Work out the finished part from the listing and answer in its coordinate system (mm). A direction names the side the tool comes from. Round coordinates to 2 decimals unless told otherwise and drop trailing zeros. Loops run counter-clockwise (first coordinate to the right, second up) from the corner with the lowest first, then second, coordinate; pieces in that order, holes last. Notation, with made-up numbers: (69.5, -35.5) - (108.5, -35.5) arc R25 cw to (108.5, -15.5) - close; hole circle Ø4 at (-29.5, 84.25). An arc over 180 degrees is marked (long way). Use CSV: the item, a comma, the result in double quotes. Start each with the question number.
from build123d import *

# Parameters (mm, degrees)
BOSS_EXTRUDE1_DEPTH      = 85
BOSS_EXTRUDE1_DEPTH_BACK = 85
SKETCH1_W                = 25
SKETCH1_H                = 25
SKETCH1_W_2              = 22
SKETCH1_H_2              = 22
SKETCH2_R                = 2
CUT_EXTRUDE1_DEPTH       = 25
SKETCH3_R                = 2
CUT_EXTRUDE2_DEPTH       = 25


with BuildPart() as part:
    # Sketch1 → Boss-Extrude1 (new, two sides: drawn at the far end of the back side and taken through both)
    with BuildSketch(Plane(origin=(0, 0, 0), x_dir=(1, 0, 0), z_dir=(0, 1, 0)).offset(-BOSS_EXTRUDE1_DEPTH_BACK)):
        Rectangle(SKETCH1_W, SKETCH1_H)
        Rectangle(SKETCH1_W_2, SKETCH1_H_2, mode=Mode.SUBTRACT)
    extrude(amount=BOSS_EXTRUDE1_DEPTH + BOSS_EXTRUDE1_DEPTH_BACK)

    # Sketch2 → Cut-Extrude1 (cut)
    with BuildSketch(Plane(origin=(0, 0, -12.5), x_dir=(-1, 0, 0), z_dir=(0, 0, -1))):
        with Locations((7.5, 80)):
            Circle(SKETCH2_R)
        with Locations((7.5, 70)):
            Circle(SKETCH2_R)
        with Locations((-7.5, 80)):
            Circle(SKETCH2_R)
        with Locations((-7.5, 70)):
            Circle(SKETCH2_R)
        with Locations((7.5, 60)):
            Circle(SKETCH2_R)
        with Locations((-7.5, 60)):
            Circle(SKETCH2_R)
    cut_extrude1 = extrude(amount=-CUT_EXTRUDE1_DEPTH, mode=Mode.SUBTRACT)

    # Mirror1: Cut-Extrude1 across plane
    add(cut_extrude1.mirror(Plane.ZX), mode=Mode.SUBTRACT)

    # Sketch3 → Cut-Extrude2 (cut)
    with BuildSketch(Plane(origin=(12.5, 0, 0), x_dir=(0, 0, -1), z_dir=(1, 0, 0))):
        with Locations((5.5, 53)):
            Circle(SKETCH3_R)
        with Locations((5.5, 42)):
            Circle(SKETCH3_R)
        with Locations((-5.5, 53)):
            Circle(SKETCH3_R)
        with Locations((-5.5, 42)):
            Circle(SKETCH3_R)
    extrude(amount=-CUT_EXTRUDE2_DEPTH, mode=Mode.SUBTRACT)


solid = part.part
Item 1: This flat-tipped pin is pushed along its axis until it touches: pin 1 Ø5 at (y, z) = (53, 5.5) entering from -X. Where does it stop, or does it pass through?
Item 2: A cutting plane is placed at A-A (z = 5.5). Determine the outline of the cut face in (x, y).
Item 3: Find the intervals of material crossed by probe 1 along Y at (x, z) = (-11.5, 5.5); probe 2 along X at (y, z) = (-70, -11.8); probe 3 along Z at (x, y) = (-5.5, 68), in increasing order. Write a range as [from, to].
Item 4: The mould has two halves that part along X. Classify faces 3 (the cylindrical face through (-11.74, 54.352, -4.026)), 4 (the flat face through (12.5, -1, 0)), 5 (the cylindrical face through (-7.24, -81.983, -11.76)): pulls with the +X half, pulls with the -X half, needs draft (parallel to the pull), parting line crosses it, or undercut.
Item 5: A cutting plane is placed at D-D (y = -44.5). Determine the outline of the cut face in (x, z), plus the area to 3 significant figures.
Item 6: A cutting plane is placed at C-C (x = 4). Determine the outline of the cut face in (y, z), plus the area to 3 significant figures.
Item 7: A cutting plane is placed at B-B (y = 60). Determine the outline of the cut face in (x, z), plus the area to 3 significant figures.
Item 8: Which of the six approach directions +Z, -Z, +X, -X, +Y, -Y give full straight-line access (tool end or side, diameter ignored) to faces 1 (the flat face through (-11, -1, 0)), 2 (the cylindrical face through (7.76, -71.983, -11.76))?
Result sheet:
1,pin 1,"x = -12.5"
2,outline,"(-12.5, -85) - (-11, -85) - (-11, 40) - (-12.5, 40) - close; (-12.5, 44) - (-11, 44) - (-11, 51) - (-12.5, 51) - close; (-12.5, 55) - (-11, 55) - (-11, 85) - (-12.5, 85) - close; (11, -85) - (12.5, -85) - (12.5, 40) - (11, 40) - close; (11, 44) - (12.5, 44) - (12.5, 51) - (11, 51) - close; (11, 55) - (12.5, 55) - (12.5, 85) - (11, 85) - close"
3,probe 1,"[-85, 40], [44, 51], [55, 85]"
3,probe 2,"[-12.5, -9.5], [-5.5, 5.5], [9.5, 12.5]"
3,probe 3,"[-12.5, -11], [11, 12.5]"
4,face 3,"needs draft"
4,face 4,"pulls with the +X half"
4,face 5,"undercut"
5,outline,"(-12.5, -12.5) - (12.5, -12.5) - (12.5, 12.5) - (-12.5, 12.5) - close; hole (-11, -11) - (11, -11) - (11, 11) - (-11, 11) - close"
5,area,"141 mm^2"
6,outline,"(-85, -12.5) - (85, -12.5) - (85, -11) - (-85, -11) - close; (-85, 11) - (85, 11) - (85, 12.5) - (-85, 12.5) - close"
6,area,"510 mm^2"
7,outline,"(-12.5, -12.5) - (-9.5, -12.5) - (-9.5, -11) - (-11, -11) - (-11, 11) - (-9.5, 11) - (-9.5, 12.5) - (-12.5, 12.5) - close; (-5.5, -12.5) - (5.5, -12.5) - (5.5, -11) - (-5.5, -11) - close; (-5.5, 11) - (5.5, 11) - (5.5, 12.5) - (-5.5, 12.5) - close; (9.5, -12.5) - (12.5, -12.5) - (12.5, 12.5) - (9.5, 12.5) - (9.5, 11) - (11, 11) - (11, -11) - (9.5, -11) - close"
7,area,"117 mm^2"
8,face 1,"+Y, -Y"
8,face 2,"+Z, -Z"
